Could you check a few things on this model? Use its own coordinates, in mm. A direction names the side the tool comes from. Round coordinates to 2 decimals unless told otherwise and drop trailing zeros. Write each loop counter-clockwise with the first axis right and the second up, starting at its lowest first coordinate (ties: lowest second). Pieces come first, ordered by that corner, then holes. Notation, with made-up numbers: (-16, 82.5) - (12, 82.5) arc R24 ccw to (12, 106.5) - close; hole circle Ø9 at (-39.5, 23). An arc over 180 degrees is marked (long way). Write each question's results on one line, items separated by ' | '. Start each with the question number.
(1) On a 3-axis mill with a long thin cutter (end or side, diameter ignored), from which of +Z, -Z, +X, -X, +Y, -Y can I reach the whole of each face in a straight line? I mean faces 1 (the flat face through (22.225, 13, -213)), 2 (the flat face through (24, 13, -431.8)). Say none if no direction works.
(2) Thinking about a two-plate mould opening in Y: for faces 3 (the flat face through (13, 25.4, -213)), 4 (the flat face through (3.175, 13, -213)), 5 (the flat face through (13, 0, -213)), 6 (the flat face through (25.4, 13, -213)), which applies, +Y half, -Y half, draft (parallel to the pull), parting line (faces both ways), or undercut?
(3) Please list where these lines run through material, in increasing order: line 1 (X direction, y = 6.75, z = -187) (3 decimals); line 2 (Y direction, x = 24.3, z = -342.9) (3 decimals). Write a range as [from, to].
(4) For P1, Ø10, axis at x = 12.7, z = -152.4, coming from the -Y side, with a flat end and sliding along its axis, tell me the tip position at first contact or that it passes through.
(5) Imagine slicing it at A-A on z = -310.5. Write out the boundary of the cut face in (x, y) (3 decimals).
Autodesk Inventor part; units mm, degrees
ref_plane "YZ Plane" through (0, 0, 0) normal (1, 0, 0) x (0, 1, 0)
ref_plane "XZ Plane" through (0, 0, 0) normal (0, 1, 0) x (-1, 0, 0)
ref_plane "XY Plane" through (0, 0, 0) normal (0, 0, 1) x (1, 0, 0)
sketch "Sketch1" plane through (0, 0, 0) normal (0, 0, 1) x (1, 0, 0)
  line L0 (0, 0) -> (25.4, 0)
  line L1 (25.4, 0) -> (25.4, 25.4)
  line L2 (25.4, 25.4) -> (0, 25.4)
  line L3 (0, 25.4) -> (0, 0)
  line L4 (3.175, 3.175) -> (22.225, 3.175)
  line L5 (22.225, 3.175) -> (22.225, 22.225)
  line L6 (22.225, 22.225) -> (3.175, 22.225)
  line L7 (3.175, 22.225) -> (3.175, 3.175)
  dimension "d0" = 25.4
  dimension "d1" = 25.4
  dimension "d2" = 3.175
extrude "Extrusion1" add sketch "Sketch1" against normal blind 431.8
sketch "Sketch2" plane through (0, 25.4, 0) normal (0, 1, 0) x (1, 0, 0)
  line L0 (25.4, 431.8) -> (0, 431.8)
  point P0 (12.7, 406.4)
  point P1 (12.7, 330.2)
  point P2 (12.7, 152.4)
  dimension "d5" = 25.4
  dimension "d6" = 76.2
  dimension "d7" = 177.8
hole "Hole1" at (12.7, 25.4, -406.4) at (12.7, 25.4, -330.2) at (12.7, 25.4, -152.4) direction (0, -1, 0) diameter 6.35 depth 25.4 tip angle 118
sketch "Sketch3" plane through (25.4, 0, 0) normal (1, 0, 0) x (0, 0, -1)
  line L0 (0, 0) -> (0, 25.4)
  line L1 (0, 0) -> (431.8, 0)
  line L2 (431.8, 0) -> (431.8, 25.4)
  point P0 (63.5, 12.7)
  point P1 (88.9, 12.7)
  point P2 (114.3, 12.7)
  point P3 (342.9, 12.7)
  point P4 (317.5, 12.7)
  point P5 (292.1, 12.7)
  point P6 (431.8, 12.7)
  dimension "d15" = 12.7
  dimension "d16" = 25.4
  dimension "d17" = 25.4
  dimension "d18" = 63.5
  dimension "d26" = 25.4
  dimension "d27" = 25.4
  dimension "d28" = 88.9
hole "Hole2" at (25.4, 12.7, -63.5) at (25.4, 12.7, -88.9) at (25.4, 12.7, -114.3) direction (-1, 0, 0) diameter 6.35 depth 25.4 tip angle 118
hole "Hole3" at (25.4, 12.7, -342.9) at (25.4, 12.7, -317.5) at (25.4, 12.7, -292.1) direction (-1, 0, 0) diameter 6.35 depth 25.4 tip angle 118
properties part number "12 in tube"
Response:
1) face 1: +Z, -Z | face 2: -Z, +X, -X, +Y, -Y
2) face 3: +Y half | face 4: undercut | face 5: -Y half | face 6: draft
3) line 1: [0, 3.175], [22.225, 25.4] | line 2: [0, 9.525], [15.875, 25.4]
4) P1: y = 0
5) outline: (0, 0) - (25.4, 0) - (25.4, 25.4) - (0, 25.4) - close; hole (3.175, 3.175) - (22.225, 3.175) - (22.225, 22.225) - (3.175, 22.225) - close
